Source: CAD feature listing. Evaluate the final solid. Frame: model axes, mm. Face numbers are marked on the shaded views. A direction names the side the tool comes from. Give positions to 0.01 mm unless a question says otherwise; leave off trailing zeros. Write each loop counter-clockwise with the first axis right and the second up, starting at its lowest first coordinate (ties: lowest second). Pieces come first, ordered by that corner, then holes. Notation, with made-up numbers: M 25.25,-26.5 L 75.25,-26.5 A7 cw 75.25,-18.5 Z; hole C 6.25,12 d8. An arc over 180 degrees is marked long. Use CSV: the item, a comma, the result in double quotes. Start each with the question number.
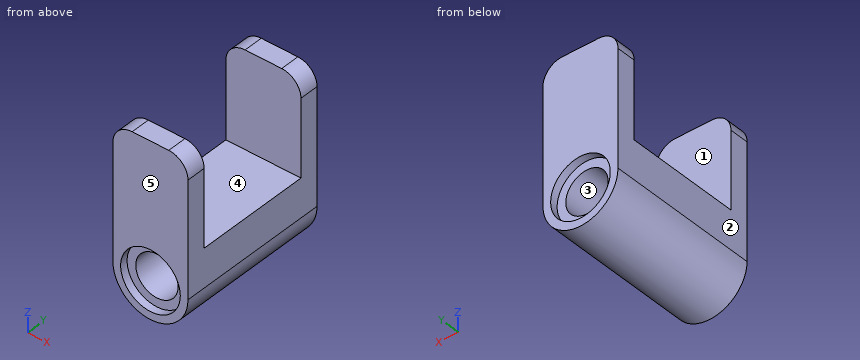
from build123d import *

# Parameters (mm, degrees)
F2_R     = 3.1
F2_R_2   = 2.2
F4_DEPTH = 8
F3_W     = 12
F3_H     = 10
F5_DEPTH = 12.5
F6_R     = 2
F7_DEPTH = 0.8


# Not quite as in the source:
# - the program builds the solid bodies; features that only make, move or delete a surface that nothing else refers to are left out


with BuildPart() as f4:
    # F2 (on Front) → F4 (new body, symmetric)
    with BuildSketch(Plane.XZ):
        with BuildLine():
            Line((3.8994949366, 10), (-3.8994949366, 10))
            Line((-3.8994949366, 10), (-3.8994949366, -4))
            ThreePointArc((-3.8994949366, -4), (0, -7.8994949366), (3.8994949366, -4))
            Line((3.8994949366, -4), (3.8994949366, 10))
        make_face()
        with Locations((0, -4)):
            Circle(F2_R, mode=Mode.SUBTRACT)
        with Locations((0, -4)):
            Circle(F2_R)
        with Locations((0, -4)):
            Circle(F2_R_2, mode=Mode.SUBTRACT)
    extrude(amount=F4_DEPTH, both=True)

    # F3 (on Right) → F5 (cut, symmetric)
    with BuildSketch(Plane.YZ):
        with Locations((0, 5)):
            Rectangle(F3_W, F3_H)
    extrude(amount=F5_DEPTH, both=True, mode=Mode.SUBTRACT)

    # F6
    f6_edges = [f4.edges().sort_by_distance(p)[0] for p in [
        (-3.899495, -7, 10),
        (3.899495, -7, 10),
        (3.899495, 7, 10),
        (-3.899495, 7, 10),
    ]]
    fillet(f6_edges, radius=F6_R)


with BuildPart() as f7:
    # F2 (on Front) → F7 (new body)
    with BuildSketch(Plane.XZ):
        with Locations((0, -4)):
            Circle(F2_R)
        with Locations((0, -4)):
            Circle(F2_R_2, mode=Mode.SUBTRACT)
    extrude(amount=F7_DEPTH)


with BuildPart() as f7_1:
    # F8: moved
    add(f7.part.moved(Location((0, 8, 0))))


with BuildPart() as f9_1:
    # F9: instance of F7
    add(f7_1.part.mirror(Plane.XZ))


with BuildPart() as f4_1:
    add(f4.part)

    # F10: cut F7, F9_1
    add(f7_1.part, mode=Mode.SUBTRACT)
    add(f9_1.part, mode=Mode.SUBTRACT)


solid = f4_1.part
Item 1: Section D-D (x = 1.25). Return the cut outline in (y, z), plus the area to 3 significant figures.
Item 2: Section C-C (y = 1). Return the cut outline in (x, z).
Item 3: Pull-direction query (Y, two-part tool) for the marked faces 3, 4 and 5; classes: released by +Y, released by -Y, zero draft, split by the parting line, or undercut.
Item 4: Contact query for a flat-ended pin moving along its axis: pin 1 Ø1 at (y, z) = (6, -5.5) entering from -X. Output: stop coordinate, or through.
Item 5: Section B-B (z = 6). Return the cut outline in (x, y).
Item 6: Section A-A (x = 0). Return the cut outline in (y, z).
Item 7: Material intervals for probe 1 along Z at (x, y) = (0, 7.5); probe 2 along Y at (x, z) = (0.5, 2.5); probe 3 along Z at (x, y) = (0, -0.5), sorted ascending.
Item 8: Set-up query: the marked faces 1 and 2. Return all of +Z, -Z, +X, -X, +Y, -Y with unobstructed straight access to the full face (end or side cutting, diameter ignored); none if empty.
Output values:
1,outline,"M -8,-7.69 L 8,-7.69 L 8,-6.84 L 7.2,-6.84 L 7.2,-5.81 L -7.2,-5.81 L -7.2,-6.84 L -8,-6.84 Z; M -8,-1.16 L -7.2,-1.16 L -7.2,-2.19 L 7.2,-2.19 L 7.2,-1.16 L 8,-1.16 L 8,10 L 6,10 L 6,0 L -6,0 L -6,10 L -8,10 Z"
1,area,"102 mm2"
2,outline,"M -3.9,-4 A3.9 ccw 3.9,-4 L 3.9,0 L -3.9,0 Z; hole C 0,-4 d4.4"
3,face 3,"zero draft"
3,face 4,"undercut"
3,face 5,"released by -Y"
4,pin 1,"stops at x = -3.77"
5,outline,"M -3.9,-8 L 3.9,-8 L 3.9,-6 L -3.9,-6 Z; M -3.9,6 L 3.9,6 L 3.9,8 L -3.9,8 Z"
6,outline,"M -8,-7.9 L 8,-7.9 L 8,-7.1 L 7.2,-7.1 L 7.2,-6.2 L -7.2,-6.2 L -7.2,-7.1 L -8,-7.1 Z; M -8,-0.9 L -7.2,-0.9 L -7.2,-1.8 L 7.2,-1.8 L 7.2,-0.9 L 8,-0.9 L 8,10 L 6,10 L 6,0 L -6,0 L -6,10 L -8,10 Z"
7,probe 1,"z = -7.9 to -7.1, -0.9 to 10"
7,probe 2,"y = -8 to -6, 6 to 8"
7,probe 3,"z = -7.9 to -6.2, -1.8 to 0"
8,face 1,"+Z, +X, -X"
8,face 2,"+Z, -Z, -X, +Y, -Y"
